```python
from build123d import *

# Parameters (mm, degrees)
BOSS_EXTRUDE4_DEPTH = 1.5
SKETCH8_W           = 6
SKETCH8_H           = 3
BOSS_EXTRUDE5_DEPTH = 1.5
BOSS_EXTRUDE6_DEPTH = 1.5


with BuildPart() as part:
    # Sketch6 → Boss-Extrude4 (new body, symmetric)
    with BuildSketch(Plane(origin=(0, 0, 0), x_dir=(1, 0, 0), z_dir=(0, 1, 0))):
        with BuildLine():
            Line((-3, 10.5), (3, 10.5))
            ThreePointArc((3, 10.5), (5.121320344, 9.621320344), (6, 7.5))
            Line((6, 7.5), (6, -7.5))
            Line((6, -7.5), (-6, -7.5))
            Line((-6, -7.5), (-6, 7.5))
            ThreePointArc((-6, 7.5), (-5.121320344, 9.621320344), (-3, 10.5))
        make_face()
    extrude(amount=BOSS_EXTRUDE4_DEPTH, both=True)

    # Sketch8 → Boss-Extrude5 (add, symmetric)
    with BuildSketch(Plane(origin=(0, 0, 0), x_dir=(1, 0, 0), z_dir=(0, 1, 0))):
        with Locations((0, -9)):
            Rectangle(SKETCH8_W, SKETCH8_H)
    extrude(amount=BOSS_EXTRUDE5_DEPTH, both=True)

    # Sketch9 → Boss-Extrude6 (add, symmetric)
    with BuildSketch(Plane(origin=(0, 0, 0), x_dir=(1, 0, 0), z_dir=(0, 1, 0))):
        Polygon((-6, -1.5), (-8, -7.5), (-6, -7.5), align=None)
        Polygon((6, -1.5), (6, -7.5), (8, -7.5), align=None)
    extrude(amount=BOSS_EXTRUDE6_DEPTH, both=True)


solid = part.part
```
Part model, mm, in its own coordinate system. A direction names the side the tool comes from. Give positions to 0.01 mm unless a question says otherwise; leave off trailing zeros. Loops run counter-clockwise (first coordinate to the right, second up) from the corner with the lowest first, then second, coordinate; pieces in that order, holes last. Notation, with made-up numbers: M 7,-15.5 L 63,-15.5 A28 cw 63,8.5 Z; hole C 49.25,53.5 d5. An arc over 180 degrees is marked long. Return JSON: item names as keys, results as strings.
1) Saw through at B-B, the plane z = -3.25. List the corners of the cut face in (x, y).
Calculated:
{"outline": "M -6,-1.5 L 6,-1.5 L 6,1.5 L -6,1.5 Z"}
2) Drill centre lines: line 1 (X direction, y = -0.6, z = 8.75); line 2 (X direction, y = 1.2, z = -4.25); line 3 (Z direction, x = -5.25, y = -0.95). Where is each one in solid material? Low to high.
Calculated:
{"line 1": "x = -3 to 3", "line 2": "x = -6 to 6", "line 3": "z = -9.48 to 7.5"}
3) Flat gauge pins, fed straight in: pin 1 Ø1.5 at (y, z) = (0, -3) entering from -X; pin 2 Ø0.9 at (x, y) = (-6.5, -0.5) entering from +Z; pin 3 Ø0.9 at (y, z) = (-0.5, 9) entering from +X. Where does each tip first touch, or does it go through?
Calculated:
{"pin 1": "stops at x = -6", "pin 2": "stops at z = 7.5", "pin 3": "stops at x = 3"}
4) Saw through at A-A, the plane y = -1.15. List the corners of the cut face in (x, z).
Calculated:
{"outline": "M -8,7.5 L -6,1.5 L -6,-7.5 A3 ccw -3,-10.5 L 3,-10.5 A3 ccw 6,-7.5 L 6,1.5 L 8,7.5 L 3,7.5 L 3,10.5 L -3,10.5 L -3,7.5 Z"}
5) 3-axis set-ups, long thin cutter, end or side, ignore diameter. For faces 1 (the face through (6, 0, -3)), 2 (the face through (-5, 0, 7.5)), 3 (the face through (-6, 0, -3)): which of +Z, -Z, +X, -X, +Y, -Y reach the whole face in a straight line?
Calculated:
{"face 1": "-Z, +X, +Y, -Y", "face 2": "+Z, -X, +Y, -Y", "face 3": "-Z, -X, +Y, -Y"}
6) Saw through at C-C, the plane x = -7. List the corners of the cut face in (y, z), then the cut area to 3 significant figures.
Calculated:
{"outline": "M -1.5,4.5 L 1.5,4.5 L 1.5,7.5 L -1.5,7.5 Z", "area": "9.00 mm2"}
